Could you check a few things on this model? Use its own coordinates, in mm. Face numbers are marked on the shaded views. A direction names the side the tool comes from. Coordinates: 2 decimals unless noted, no trailing zeros. Order: outer loops, then holes, each group sorted by start corner. A loop starts at its lowest first (then second) coordinate and runs counter-clockwise, first axis right, second up.
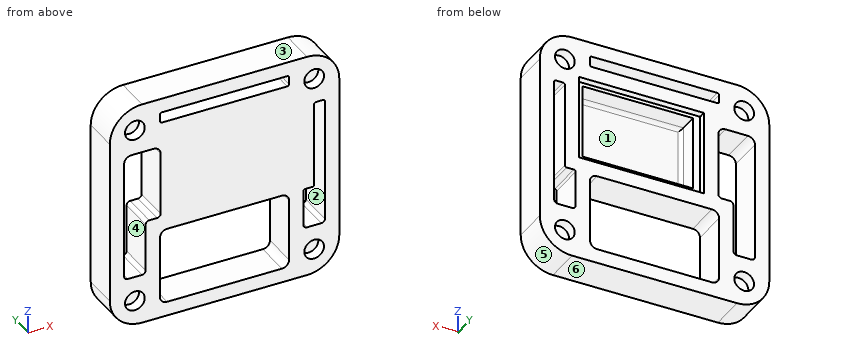
Autodesk Inventor part; units mm, degrees
ref_plane "Work Plane7" through (0, 5, 0) normal (0, 1, 0) x (1, 0, 0)
ref_plane "YZ Plane" through (0, 0, 0) normal (1, 0, 0) x (0, 1, 0)
ref_plane "XZ Plane" through (0, 0, 0) normal (0, 1, 0) x (-1, 0, 0)
sketch "Sketch1" plane through (0, 0, 0) normal (0, 1, 0) x (-1, 0, 0)
  line L0 (30, 30) -> (-30, 30)
  line L1 (-30, 30) -> (-30, -30)
  line L2 (-30, -30) -> (30, -30)
  line L3 (30, -30) -> (30, 30)
  line L4 (30, 30) -> (-30, -30) construction
  line L5 (-30, 30) -> (30, -30) construction
  point P0 (0, 0)
  dimension "d0" = 60
  dimension "d1" = 60
extrude "Extrusion1" add sketch "Sketch1" along normal blind 10
fillet "Fillet1" radius 7 4 edges at (30, 5, 30) (30, 5, -30) (-30, 5, 30) (-30, 5, -30)
sketch "Sketch2" plane through (0, 10, 0) normal (0, 1, 0) x (1, 0, 0)
  line L0 (-30, 30) -> (30, 30)
  line L1 (30, 30) -> (30, -30)
  line L2 (30, -30) -> (-30, -30)
  line L3 (-30, -30) -> (-30, 30)
  line L4 (-30, 30) -> (30, -30) construction
  line L5 (30, 30) -> (-30, -30) construction
  line L6 (25, -25) -> (25, 25)
  line L7 (25, 25) -> (-25, 25)
  line L8 (-25, 25) -> (-25, -25)
  line L9 (-25, -25) -> (25, -25)
  circle A0 centre (25, -25) radius 2.75
  circle A1 centre (-25, -25) radius 2.75
  circle A2 centre (25, 25) radius 2.75
  circle A3 centre (-25, 25) radius 2.75
  point P0 (0, 0)
  dimension "d5" = 5
  dimension "d6" = 5.5
  dimension "d7" = 5.5
  dimension "d8" = 5.5
  dimension "d9" = 5.5
extrude "Extrusion2" cut sketch "Sketch2" against normal blind 3 contours L9 A0 L6 | L6 A0 L9 | A2 L7 L6 | L6 L7 A2 | A1 L8 L9 | L9 L8 A1 | A3 L8 L7 | L7 L8 A3
sketch "Sketch7" plane through (0, 10, 0) normal (0, 1, 0) x (1, 0, 0)
  line L0 (-23, 30) -> (23, 30)
  line L1 (30, 23) -> (30, -23)
  line L2 (23, -30) -> (-23, -30)
  line L3 (-30, -23) -> (-30, 23)
  line L4 (-30, 30) -> (30, -30) construction
  line L5 (30, 30) -> (-30, -30) construction
  arc A0 (-23, 30) -> (-30, 23) centre (-23, 23) ccw
  arc A1 (-30, -23) -> (-23, -30) centre (-23, -23) ccw
  arc A2 (23, -30) -> (30, -23) centre (23, -23) ccw
  arc A3 (30, 23) -> (23, 30) centre (23, 23) ccw
  line L6 (23, 32) -> (-23, 32)
  arc A4 (-23, 32) -> (-32, 23) centre (-23, 23) ccw
  line L7 (-32, 23) -> (-32, -23)
  arc A5 (-32, -23) -> (-23, -32) centre (-23, -23) ccw
  line L8 (-23, -32) -> (23, -32)
  arc A6 (23, -32) -> (32, -23) centre (23, -23) ccw
  line L9 (32, -23) -> (32, 23)
  arc A7 (32, 23) -> (23, 32) centre (23, 23) ccw
  point P0 (0, 0)
  dimension "d47" = 7
  dimension "d48" = 2
extrude "Extrusion6" add sketch "Sketch7" against normal blind 10
sketch "Sketch27" plane through (0, 10, 0) normal (0, 1, 0) x (1, 0, 0)
  line L0 (-25, 25) -> (25, 25)
  line L1 (25, 25) -> (25, -25)
  line L2 (25, -25) -> (-25, -25)
  line L3 (-25, -25) -> (-25, 25)
  line L4 (-25, 25) -> (25, -25) construction
  line L5 (25, 25) -> (-25, -25) construction
  line L6 (21, -21) -> (21, 21)
  line L7 (21, 21) -> (-21, 21)
  line L8 (-21, 21) -> (-21, -21)
  line L9 (-21, -21) -> (21, -21)
  line L10 (-13.8, -21) -> (-13.8, 2.6)
  line L11 (21, 2.6) -> (-13.8, 2.6)
  line L12 (19, 0.6) -> (-11.8, 0.6)
  line L13 (-11.8, 0.6) -> (-11.8, -20)
  line L14 (-19, -19) -> (-19, 19)
  line L15 (-19, 19) -> (19, 19)
  line L16 (20, 20) -> (20, 0.6)
  line L17 (-20, -20) -> (-20, 20)
  line L18 (-20, 20) -> (20, 20)
  line L19 (-13.8, -19) -> (-19, -19)
  line L20 (19, -20) -> (-11.8, -20)
  line L21 (-13.8, -20) -> (-20, -20)
  line L22 (19, 19) -> (19, 2.6)
  line L23 (19, 0.6) -> (19, -20)
  point P0 (0, 0)
  dimension "d266" = 50
  dimension "d267" = 50
  dimension "d268" = 4
  dimension "d269" = 34.8
  dimension "d270" = 23.6
  dimension "d271" = 2
  dimension "d273" = 1
extrude "Extrusion25" cut sketch "Sketch27" against normal blind 2 contours L9 L10 L11 L6
sketch "Sketch28" plane through (0, 10, 0) normal (0, 1, 0) x (1, 0, 0)
  line L0 (-11.8, 0.6) -> (19, 0.6)
  line L1 (19, 0.6) -> (19, -20)
  line L2 (19, -20) -> (-11.8, -20)
  line L3 (-11.8, -20) -> (-11.8, 0.6)
  point P0 (0, 0)
extrude "Extrusion26" cut sketch "Sketch28" against normal blind 8
sketch "Sketch29" plane through (0, 10, 0) normal (0, 1, 0) x (1, 0, 0)
  line L0 (23, 32) -> (-23, 32)
  line L1 (-32, 23) -> (-32, -23)
  line L2 (32, -23) -> (32, 23)
  line L3 (-13.8, 2.6) -> (21, 2.6)
  line L4 (-18, 28) -> (18, 28)
  line L5 (18, 28) -> (18, 6.6)
  line L6 (18, 6.6) -> (-18, 6.6)
  line L7 (-18, 6.6) -> (-18, 28)
  line L8 (-23, -32) -> (23, -32)
  line L9 (21, 2.6) -> (21, -21)
  line L10 (28, 18) -> (22, 18)
  line L11 (22, 18) -> (22, 6.6)
  line L12 (22, 6.6) -> (25, 6.6)
  line L13 (28, 18) -> (28, -18)
  line L14 (28, -18) -> (25, -18)
  line L15 (25, -18) -> (25, 2.6)
  line L16 (25, 2.6) -> (25, 6.6)
  line L17 (21, -21) -> (-13.8, -21)
  line L18 (18, -28) -> (18, -25)
  line L19 (18, -25) -> (-18, -25)
  line L20 (-18, -25) -> (-18, -28)
  line L21 (-18, -28) -> (18, -28)
  line L22 (-13.8, -21) -> (-13.8, 2.6)
  line L23 (-28, -18) -> (-17.8, -18)
  line L24 (-17.8, -18) -> (-17.8, 2.6)
  line L25 (-17.8, 2.6) -> (-22, 2.6)
  line L26 (-22, 2.6) -> (-22, 6.6)
  line L27 (-28, 18) -> (-22, 18)
  line L28 (-22, 18) -> (-22, 6.6)
  line L29 (-28, 18) -> (-28, -18)
  point P0 (0, 0)
  dimension "d278" = 4
  dimension "d279" = 4
  dimension "d280" = 14
  dimension "d281" = 14
  dimension "d282" = 4
  dimension "d283" = 4
  dimension "d284" = 4
  dimension "d285" = 14
  dimension "d286" = 14
  dimension "d287" = 4
  dimension "d288" = 4
  dimension "d289" = 4
  dimension "d290" = 4
  dimension "d291" = 14
  dimension "d292" = 14
  dimension "d293" = 4
  dimension "d294" = 14
  dimension "d295" = 14
  dimension "d296" = 4
  dimension "d297" = 4
  dimension "d298" = 4
  dimension "d299" = 4
  dimension "d300" = 14
  dimension "d301" = 4
extrude "Extrusion27" cut sketch "Sketch29" against normal through all contours L4 L5 L6 L7 | L13 L14 L15 L16 L12 L11 L10 | L21 L20 L19 L18 | L29 L27 L28 L26 L25 L24 L23
ref_plane "Work Plane7" through (0, 5, 0) normal (0, 1, 0) x (1, 0, 0)
mirror "Mirror7" about plane through (0, 5, 0) normal (0, 1, 0) of "Extrusion2"
fillet "Fillet8" radius 2 6 edges at (18, 5, -28) (-18, 5, -28) (-18, 5, -6.6) (18, 5, -6.6) (-17.8, 5, 18) (-28, 5, 18)
fillet "Fillet8" radius 1 10 edges at (-28, 5, -18) (-22, 5, -18) (-22, 5, -2.6) (-17.8, 5, -2.6) (3.6, 2, -0.6) (19, 2, 9.7) (-11.8, 2, 9.7) (3.6, 2, 20) (28, 5, -18) (22, 5, -18)
fillet "Fillet8" radius 0.5 8 edges at (-18, 5, 28) (25, 5, 18) (25, 5, -6.6) (22, 5, -6.6) (28, 5, 18) (18, 5, 28) (18, 5, 25) (-18, 5, 25)
properties part number "14 pin shortest holder"
Item 1: For pin 1 Ø3.5 at (x, z) = (-25, -25) entering from -Y; pin 2 Ø3 at (x, y) = (25, 3) entering from +Z; pin 3 Ø12 at (x, z) = (4.5, 14.5) entering from +Y, each with a flat end and sliding along its axis, tell me the tip position at first contact or that it passes through.
Item 2: Suppose I cut it at C-C (x = -24). List the corners of the cut face in (y, z) for me, and give its area (3 significant figures).
Item 3: Suppose I cut it at A-A (x = -6.5). List the corners of the cut face in (y, z) for me.
Item 4: Thinking about a two-plate mould opening in X: for the marked faces 4, 5 and 6, which applies, +X half, -X half, draft (parallel to the pull), parting line (faces both ways), or undercut?
Item 5: Suppose I cut it at D-D (y = 5.25). Count the separate pieces of the cut face and the enclosed holes in it, and give its area (3 significant figures).
Item 6: Suppose I cut it at B-B (z = 2.5). List the corners of the cut face in (x, y) for me, and give its area (3 significant figures).
Item 7: Which directions (+Z, -Z, +X, -X, +Y, -Y) give clear straight access to the entire face, cutting with the end or side of a thin tool? Please do the marked faces 1, 2 and 3.
Item 8: I need wall thicknesses on line 1 (X direction, y = 7.75, z = 11); line 2 (X direction, y = 8.5, z = -17); line 3 (Z direction, x = 12, y = 1). Which ranges of each line are inside material? Lowest first, please.
Geometry results:
1. pin 1: stops at y = 3
1. pin 2: stops at z = 31.99
1. pin 3: stops at y = 8
2. outline: (0, -31.94) - (10, -31.94) - (10, -27.56) - (7, -27.56) - (7, -22.44) - (10, -22.44) - (10, -18) - (0, -18) - (0, -22.44) - (3, -22.44) - (3, -27.56) - (0, -27.56) - close; (0, 18) - (10, 18) - (10, 22.44) - (7, 22.44) - (7, 27.56) - (10, 27.56) - (10, 31.94) - (0, 31.94) - (0, 27.56) - (3, 27.56) - (3, 22.44) - (0, 22.44) - close
2. area: 217 mm2
3. outline: (0, -32) - (10, -32) - (10, -28) - (0, -28) - close; (0, -6.6) - (10, -6.6) - (10, -2.6) - (8, -2.6) - (8, -0.6) - (3, -0.6) arc R1 cw to (2, 0.4) - (2, 19) arc R1 cw to (3, 20) - (8, 20) - (8, 21) - (10, 21) - (10, 25) - (0, 25) - close; (0, 28) - (10, 28) - (10, 32) - (0, 32) - close
4. face 4: undercut
4. face 5: +X half
4. face 6: draft
5. separate pieces: 1
5. enclosed holes: 5
5. area: 2,080 mm2
6. outline: (-32, 0) - (-28, 0) - (-28, 10) - (-32, 10) - close; (-17.8, 0) - (25, 0) - (25, 10) - (21, 10) - (21, 8) - (19, 8) - (19, 3) arc R1 cw to (18, 2) - (-10.8, 2) arc R1 cw to (-11.8, 3) - (-11.8, 8) - (-13.8, 8) - (-13.8, 10) - (-17.8, 10) - close; (28, 0) - (32, 0) - (32, 10) - (28, 10) - close
6. area: 254 mm2
7. face 1: +Y
7. face 2: +Y, -Y
7. face 3: +Z, +X, -X, +Y, -Y
8. line 1: x = -32 to -28, -17.8 to -11.8, 19 to 25, 28 to 32
8. line 2: x = -32 to -28, -22 to -18, 18 to 22, 28 to 32
8. line 3: z = -32 to -28, -6.6 to 25, 28 to 32
